Check sheet for the modelled part. Datum: model origin and axes. Units: mm. Face numbers are marked on the shaded views. A direction names the side the tool comes from. Round coordinates to 2 decimals unless told otherwise and drop trailing zeros. Order: outer loops, then holes, each group sorted by start corner. A loop starts at its lowest first (then second) coordinate and runs counter-clockwise, first axis right, second up.
(1) Mould release check, pull along X, two halves, no side actions. Record for the marked faces 3, 4 and 5: released by +X, released by -X, zero draft, split by the parting line, or undercut.
(2) Tool access check on the marked faces 1 and 2. Record the directions out of +Z, -Z, +X, -X, +Y, -Y that give a thin tool (end or side, any length) a straight path to the whole face; none if there is none.
(3) Sectioned sample at A-A, the plane z = 0. Enter the section's corners in (x, y).
(4) Thickness scan on probe 1 along Z at (x, y) = (0, 0.25); probe 2 along Z at (x, y) = (0, 2.65). Record the ranges inside material, lowest first.
(5) Sectioned sample at B-B, the plane x = 0. Enter the section's corners in (y, z).
(6) Sectioned sample at C-C, the plane y = -2.5. Enter the section's corners in (x, z), and give its area (3 significant figures).
(7) Depth check by flat-ended pin: pin 1 (1.5 mm diameter, centred on x = -2.5, y = -0.5, fed in from +Z); pin 2 (4.5 mm diameter, centred on x = 0, z = 0, fed in from +Y); pin 3 (1 mm diameter, centred on y = 0, z = 2, fed in from +X); pin 4 (3 mm diameter, centred on y = -2.5, z = 2, fed in from -X). Enter the tip coordinate at first touch or a pass-through.
(8) Sectioned sample at D-D, the plane z = 2.75. Enter the section's corners in (x, y), and give its area (3 significant figures).
```python
from build123d import *

# Parameters (mm, degrees)
SKETCH_1_R          = 5.35
SKETCH_1_R_2        = 4
EXTRUDE_1_DEPTH     = 3
SKETCH_2_R          = 5.35
SKETCH_2_R_2        = 4
EXTRUDE_2_DEPTH     = 5
SKETCH_3_R          = 4
EXTRUDE_3_DEPTH     = 1
SKETCH_4_R          = 2.5
CUT_EXTRUDE_1_DEPTH = 1


with BuildPart() as part:
    # 草图1 → 凸台-拉伸1 (new body)
    with BuildSketch(Plane(origin=(0, 0, 0), x_dir=(1, 0, 0), z_dir=(0, 1, 0))):
        Circle(SKETCH_1_R)
        Circle(SKETCH_1_R_2, mode=Mode.SUBTRACT)
    extrude(amount=EXTRUDE_1_DEPTH)

    # 草图2 → 凸台-拉伸2 (add)
    with BuildSketch(Plane.XZ):
        Circle(SKETCH_2_R)
        Circle(SKETCH_2_R_2, mode=Mode.SUBTRACT)
    extrude(amount=EXTRUDE_2_DEPTH)

    # 草图3 → 凸台-拉伸3 (add)
    with BuildSketch(Plane(origin=(0, 3, 0), x_dir=(1, 0, 0), z_dir=(0, 1, 0))):
        Circle(SKETCH_3_R)
    extrude(amount=-EXTRUDE_3_DEPTH)

    # 草图4 → 切除-拉伸1 (cut)
    with BuildSketch(Plane(origin=(0, 3, 0), x_dir=(1, 0, 0), z_dir=(0, 1, 0))):
        Circle(SKETCH_4_R)
    extrude(amount=-CUT_EXTRUDE_1_DEPTH, mode=Mode.SUBTRACT)


solid = part.part
```
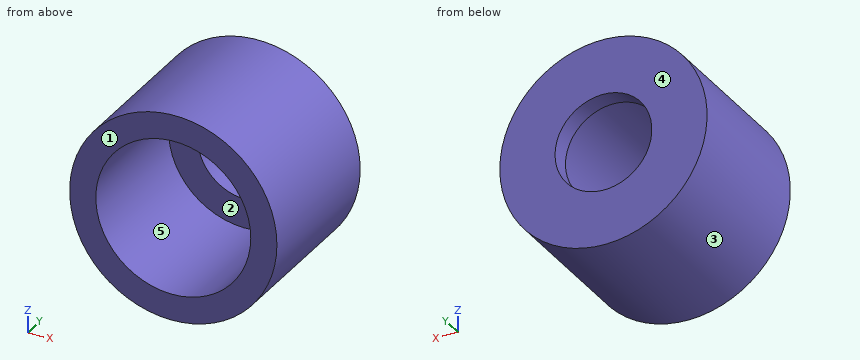
Derived:
1. face 3: split by the parting line
1. face 4: zero draft
1. face 5: undercut
2. face 1: +Z, -Z, +X, -X, -Y
2. face 2: -Y
3. outline: (-5.35, -5) - (-4, -5) - (-4, 2) - (-2.5, 2) - (-2.5, 3) - (-5.35, 3) - close; (2.5, 2) - (4, 2) - (4, -5) - (5.35, -5) - (5.35, 3) - (2.5, 3) - close
4. probe 1: z = -5.35 to -4, 4 to 5.35
4. probe 2: z = -5.35 to -2.5, 2.5 to 5.35
5. outline: (-5, -5.35) - (3, -5.35) - (3, -2.5) - (2, -2.5) - (2, -4) - (-5, -4) - close; (-5, 4) - (2, 4) - (2, 2.5) - (3, 2.5) - (3, 5.35) - (-5, 5.35) - close
6. outline: circle Ø10.7 at (0, 0); hole circle Ø8 at (0, 0)
6. area: 39.7 mm2
7. pin 1: stops at z = 5.06
7. pin 2: passes through
7. pin 3: stops at x = 5.14
7. pin 4: stops at x = -5.33
8. outline: (-4.59, -5) - (-2.9, -5) - (-2.9, 2) - (2.9, 2) - (2.9, -5) - (4.59, -5) - (4.59, 3) - (-4.59, 3) - close
8. area: 32.8 mm2
